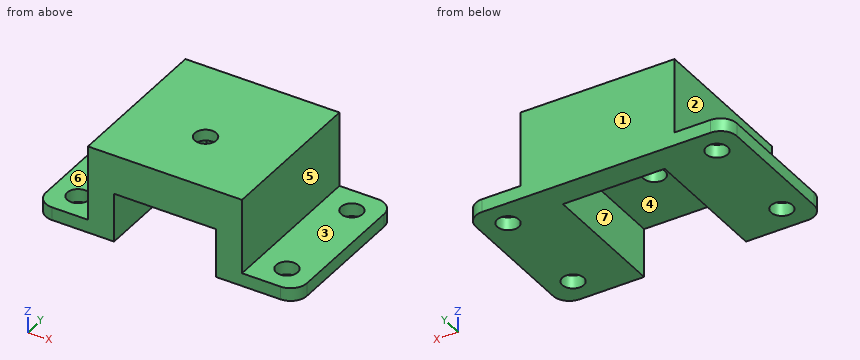
```python
from build123d import *

# Parameters (mm, degrees)
SKETCH1_R           = 1.65
BOSS_EXTRUDE1_DEPTH = 2
BOSS_EXTRUDE2_DEPTH = 5.5
SKETCH3_W           = 23.6
SKETCH3_H           = 24
SKETCH3_R           = 1.65
BOSS_EXTRUDE3_DEPTH = 6
CUT_EXTRUDE1_START  = -1.7
CUT_EXTRUDE1_DEPTH  = 2.6
FILLET1_R           = 2.5


with BuildPart() as part:
    # Sketch1 → Boss-Extrude1 (new body)
    with BuildSketch(Plane(origin=(0, 0, 0), x_dir=(0, 1, 0), z_dir=(0, 0, 1))):
        Polygon((-24, 12.4), (-4, 12.4), (-4, 28), (-24, 28), (-24, 40), (0, 40), (0, 0), (-24, 0), align=None)
        with Locations((-20, 4)):
            Circle(SKETCH1_R, mode=Mode.SUBTRACT)
        with Locations((-4, 4)):
            Circle(SKETCH1_R, mode=Mode.SUBTRACT)
        with Locations((-4, 36)):
            Circle(SKETCH1_R, mode=Mode.SUBTRACT)
        with Locations((-20, 36)):
            Circle(SKETCH1_R, mode=Mode.SUBTRACT)
    extrude(amount=BOSS_EXTRUDE1_DEPTH)

    # Sketch2 → Boss-Extrude2 (add)
    with BuildSketch(Plane.XY.offset(2)):
        Polygon((-28, -24), (-28, -4), (-12.4, -4), (-12.4, -24), (-8.4, -24), (-8.4, 0), (-32, 0), (-32, -24), align=None)
    extrude(amount=BOSS_EXTRUDE2_DEPTH)

    # Sketch3 → Boss-Extrude3 (add)
    with BuildSketch(Plane.XY.offset(7.5)):
        with Locations((-20.2, -12)):
            Rectangle(SKETCH3_W, SKETCH3_H)
        with Locations((-20.2, -14)):
            Circle(SKETCH3_R, mode=Mode.SUBTRACT)
    extrude(amount=BOSS_EXTRUDE3_DEPTH)

    # Sketch4 → Cut-Extrude1 (cut)
    with BuildSketch(Plane.XY.offset(13.5).offset(CUT_EXTRUDE1_START)):
        Polygon((-16.851368439, -14), (-18.525684219, -11.1), (-21.874315781, -11.1), (-23.548631561, -14), (-21.874315781, -16.9), (-18.525684219, -16.9), align=None)
    extrude(amount=-CUT_EXTRUDE1_DEPTH, mode=Mode.SUBTRACT)

    # Fillet1
    fillet1_edges = [part.edges().sort_by_distance(p)[0] for p in [
        (0, 0, 1),
        (0, -24, 1),
        (-40, -24, 1),
        (-40, 0, 1),
    ]]
    fillet(fillet1_edges, radius=FILLET1_R)


solid = part.part
```
Can you work these out from the model? Positions are in its coordinate system, mm. Face numbers are marked on the shaded views. A direction names the side the tool comes from. Coordinates: 2 decimals unless noted, no trailing zeros. Loops run counter-clockwise (first coordinate to the right, second up) from the corner with the lowest first, then second, coordinate; pieces in that order, holes last. Notation, with made-up numbers: M 81.25,12 L 93.25,12 A29 ccw 93.25,37 Z; hole C 70.5,-27.75 d9. An arc over 180 degrees is marked long. Put each result on its own line as item: value. Start each with the question number.
(1) Which directions (+Z, -Z, +X, -X, +Y, -Y) give clear straight access to the entire face, cutting with the end or side of a thin tool? Please do the marked faces 1, 2, 3 and 4.
(2) Imagine slicing it at C-C on x = -36. List the corners of the cut face in (y, z) for me.
(3) I need wall thicknesses on probe 1 along Y at (x, z) = (-4, 0.65); probe 2 along X at (y, z) = (-20, 1.2); probe 3 along X at (y, z) = (-14, 8.2). Which ranges of each line are inside material? Lowest first, please.
(4) We'd pull the mould along X, two halves only. Please class the marked faces 5, 6 and 7: +X half, -X half, draft (parallel to the pull), parting line (faces both ways), or undercut.
(5) Imagine slicing it at A-A on y = -20. List the corners of the cut face in (x, z) for me.
(6) Imagine slicing it at D-D on y = -9.5. List the corners of the cut face in (x, z) for me.
(7) Imagine slicing it at B-B on z = 10.25. List the corners of the cut face in (x, y) for me.
(8) Will these pins go through, and if not, where does the flat tip stop? pin 1 Ø2 at (x, y) = (-36, -20) entering from +Z; pin 2 Ø3 at (x, y) = (-20.5, -14.5) entering from -Z; pin 3 Ø3 at (x, y) = (-36, -12) entering from +Z; pin 4 Ø6 at (y, z) = (-16, 9) entering from +X.
Worked answers:
1. face 1: +Z, -Z, +X, -X, +Y
1. face 2: +Z, -X, +Y, -Y
1. face 3: +Z, +X, +Y, -Y
1. face 4: -Z, -Y
2. outline: M -24,0 L -21.65,0 L -21.65,2 L -24,2 Z; M -18.35,0 L -5.65,0 L -5.65,2 L -18.35,2 Z; M -2.35,0 L 0,0 L 0,2 L -2.35,2 Z
3. probe 1: y = -24 to -21.65, -18.35 to -5.65, -2.35 to 0
3. probe 2: x = -40 to -37.65, -34.35 to -28, -12.4 to -5.65, -2.35 to 0
3. probe 3: x = -32 to -21.85, -18.55 to -8.4
4. face 5: +X half
4. face 6: draft
4. face 7: undercut
5. outline: M -40,0 L -37.65,0 L -37.65,2 L -40,2 Z; M -34.35,0 L -28,0 L -28,7.5 L -12.4,7.5 L -12.4,0 L -5.65,0 L -5.65,2 L -8.4,2 L -8.4,13.5 L -32,13.5 L -32,2 L -34.35,2 Z; M -2.35,0 L 0,0 L 0,2 L -2.35,2 Z
6. outline: M -40,0 L -28,0 L -28,7.5 L -12.4,7.5 L -12.4,0 L 0,0 L 0,2 L -8.4,2 L -8.4,13.5 L -32,13.5 L -32,2 L -40,2 Z
7. outline: M -32,-24 L -8.4,-24 L -8.4,0 L -32,0 Z; hole M -23.55,-14 L -21.87,-16.9 L -18.53,-16.9 L -16.85,-14 L -18.53,-11.1 L -21.87,-11.1 Z
8. pin 1: passes through
8. pin 2: stops at z = 7.5
8. pin 3: stops at z = 2
8. pin 4: stops at x = -8.4
